from build123d import *

# Parameters (mm, degrees)
SKETCH1_W               = 385
SKETCH1_H               = 25
SKETCH1_W_2             = 125
BOSS_EXTRUDE4_DEPTH     = 25
FILLET1_R               = 10
FILLET2_R               = 10
SKETCH8_W               = 50
SKETCH8_H               = 50
SKETCH8_W_2             = 40
SKETCH8_H_2             = 40
BOSS_EXTRUDE5_DEPTH     = 280
CUT_EXTRUDE2_DEPTH      = 51
CUT_EXTRUDE2_DEPTH_BACK = 626.028762059
SKETCH11_R              = 7
SKETCH12_R              = 7
CUT_EXTRUDE3_DEPTH      = 1112.711398879
SKETCH13_R              = 12.5
CUT_EXTRUDE4_DEPTH      = 25


with BuildPart() as part:
    # Sketch1 → Boss-Extrude4 (new, symmetric)
    with BuildSketch(Plane.XY):
        Polygon((-254.98711306, -118.349364905), (-242.48711306, -140), (0, 0), (265, 0), (265, 25), (-6.698729811, 25), align=None)
        Polygon((0, 0), (-242.48711306, -140), (-229.98711306, -161.650635095), (6.698729811, -25), (775, -25), (775, 0), (650, 0), (265, 0), align=None)
        with Locations((457.5, 12.5)):
            Rectangle(SKETCH1_W, SKETCH1_H)
        with Locations((712.5, 12.5)):
            Rectangle(SKETCH1_W_2, SKETCH1_H)
    extrude(amount=BOSS_EXTRUDE4_DEPTH, both=True)

    # Fillet1
    fillet1_edges = [part.edges().sort_by_distance(p)[0] for p in [
        (-6.698729811, 25, 0),
    ]]
    fillet(fillet1_edges, radius=FILLET1_R)

    # Fillet2
    fillet2_edges = [part.edges().sort_by_distance(p)[0] for p in [
        (6.698729811, -25, 0),
    ]]
    fillet(fillet2_edges, radius=FILLET2_R)

    # Sketch8 → Boss-Extrude5 (add)
    # profile 1 of 2: a face of its own
    with BuildSketch(Plane(origin=(0, 25, 0), x_dir=(1, 0, 0), z_dir=(0, 1, 0))):
        with Locations((265, 0)):
            Rectangle(SKETCH8_W, SKETCH8_H)
        with Locations((265, 0)):
            Rectangle(SKETCH8_W_2, SKETCH8_H_2, mode=Mode.SUBTRACT)
    # profile 2 of 2: a face of its own
    with BuildSketch(Plane(origin=(0, 25, 0), x_dir=(1, 0, 0), z_dir=(0, 1, 0))):
        with Locations((650.033558731, 0)):
            Rectangle(SKETCH8_W, SKETCH8_H)
        with Locations((650.033558731, 0)):
            Rectangle(SKETCH8_W_2, SKETCH8_H_2, mode=Mode.SUBTRACT)
    extrude(amount=BOSS_EXTRUDE5_DEPTH)

    # Sketch11 → Cut-Extrude2 (cut, two sides: drawn at the far end of the back side and taken through both)
    with BuildSketch(Plane(origin=(290, 0, 0), x_dir=(0, 0, -1), z_dir=(1, 0, 0)).offset(-CUT_EXTRUDE2_DEPTH_BACK)):
        with Locations((0, 260)):
            Circle(SKETCH11_R)
    extrude(amount=CUT_EXTRUDE2_DEPTH + CUT_EXTRUDE2_DEPTH_BACK, mode=Mode.SUBTRACT)

    # Mirror1: part across plane


with BuildPart() as part_1:
    add(part.part)
    add(part.part.mirror(Plane(origin=(0, 305, 0), x_dir=(0, 0, 1), z_dir=(0, -1, 0))))

    # Sketch12 → Cut-Extrude3 (cut, through all)
    with BuildSketch(Plane.XZ.offset(25)):
        with Locations(Location((310, 0, 0), (0, 0, 270))):
            Circle(SKETCH12_R)
        with Locations(Location((220, 0, 0), (0, 0, 270))):
            Circle(SKETCH12_R)
        with Locations(Location((597.5, 0, 0), (0, 0, 270))):
            Circle(SKETCH12_R)
        with Locations(Location((702.5, 0, 0), (0, 0, 270))):
            Circle(SKETCH12_R)
    extrude(amount=-CUT_EXTRUDE3_DEPTH, mode=Mode.SUBTRACT)

    # Sketch13 → Cut-Extrude4 (cut)
    with BuildSketch(Plane.XY.offset(25)):
        with Locations((265, 395)):
            Circle(SKETCH13_R)
        with Locations(Location((265, 215, 0), (0, 0, 180))):
            Circle(SKETCH13_R)
    extrude(amount=-CUT_EXTRUDE4_DEPTH, mode=Mode.SUBTRACT)


solid = part_1.part
Read the model definition and answer for the solid it produces. Units are mm, in the model's axes. A direction names the side the tool comes from. Give positions to 0.01 mm unless a question says otherwise; leave off trailing zeros. Write each loop counter-clockwise with the first axis right and the second up, starting at its lowest first coordinate (ties: lowest second). Pieces come first, ordered by that corner, then holes. Notation, with made-up numbers: (76.25, 27.25) - (104.25, 27.25) arc R15 ccw to (104.25, 38.25) - close; hole circle Ø8 at (26, 83.25). An arc over 180 degrees is marked (long way). Return JSON: item names as keys, results as strings.
Q1. A cutting plane is placed at C-C, the plane x = 567. Determine the outline of the cut face in (y, z).
Reply:
{"outline": "(-25, -25) - (25, -25) - (25, 25) - (-25, 25) - close; (585, -25) - (635, -25) - (635, 25) - (585, 25) - close"}
Q2. A cutting plane is placed at A-A, the plane y = 215. Determine the outline of the cut face in (x, z).
Reply:
{"outline": "(240, -25) - (290, -25) - (290, 25) - (277.5, 25) - (277.5, 20) - (285, 20) - (285, -20) - (245, -20) - (245, 20) - (252.5, 20) - (252.5, 25) - (240, 25) - close; (625.03, -25) - (675.03, -25) - (675.03, 25) - (625.03, 25) - close; hole (630.03, -20) - (670.03, -20) - (670.03, 20) - (630.03, 20) - close"}
Q3. For faces 4 (the face through (240, 309, 0)), 5 (the face through (460, 25, 0)), 6 (the face through (265, 585, 0)), determine the directions among +Z, -Z, +X, -X, +Y, -Y from which every point of the face is accessible in a straight line to the end or side of a thin tool.
Reply:
{"face 4": "+Z, -Z, -X", "face 5": "+Z, -Z", "face 6": "none"}
Q4. Given P1, Ø8.5, axis at x = 702.5, z = 0, coming from the +Y side; P2, Ø25, axis at x = 749, z = 9, coming from the +Y side; P3, Ø3, axis at y = 422, z = -11, coming from the +X side; P4, Ø15, axis at y = 250.5, z = 11, coming from the -X side, each flat-ended and moving along its own axis, determine where each tip first touches the part or whether it passes through.
Reply:
{"P1": "through", "P2": "y = 635", "P3": "x = 675.03", "P4": "x = 240"}
Q5. A cutting plane is placed at B-B, the plane y = 64.5. Determine the outline of the cut face in (x, z), and give its area (3 significant figures).
Reply:
{"outline": "(240, -25) - (290, -25) - (290, 25) - (240, 25) - close; (625.03, -25) - (675.03, -25) - (675.03, 25) - (625.03, 25) - close; hole (245, -20) - (285, -20) - (285, 20) - (245, 20) - close; hole (630.03, -20) - (670.03, -20) - (670.03, 20) - (630.03, 20) - close", "area": "1,800 mm²"}
Q6. For a pull along Y with two mould halves and no side action, classify faces 1 (the face through (-242.66, 749.7, 0.35)), 2 (the face through (775, 610, 0)), 3 (the face through (290, 309, 0)) as released by +Y, released by -Y, zero draft, split by the parting line, or undercut.
Reply:
{"face 1": "released by +Y", "face 2": "zero draft", "face 3": "undercut"}
Q7. A cutting plane is placed at D-D, the plane x = 265. Determine the outline of the cut face in (y, z).
Reply:
{"outline": "(-25, -25) - (635, -25) - (635, 25) - (407.5, 25) - (407.5, 20) - (585, 20) - (585, -20) - (25, -20) - (25, 20) - (202.5, 20) - (202.5, 25) - (-25, 25) - close; (227.5, 20) - (382.5, 20) - (382.5, 25) - (227.5, 25) - close"}
Q8. Consider line 1 along X through (y, z) = (479, -19); line 2 along X through (y, z) = (284.5, -21); line 3 along Z through (x, y) = (286.7, 350). Determine where each line is inside the solid, lowest interval first. Write a range as [from, to].
Reply:
{"line 1": "[240, 245], [285, 290], [625.03, 630.03], [670.03, 675.03]", "line 2": "[240, 290], [625.03, 675.03]", "line 3": "[-25, -7], [7, 25]"}
